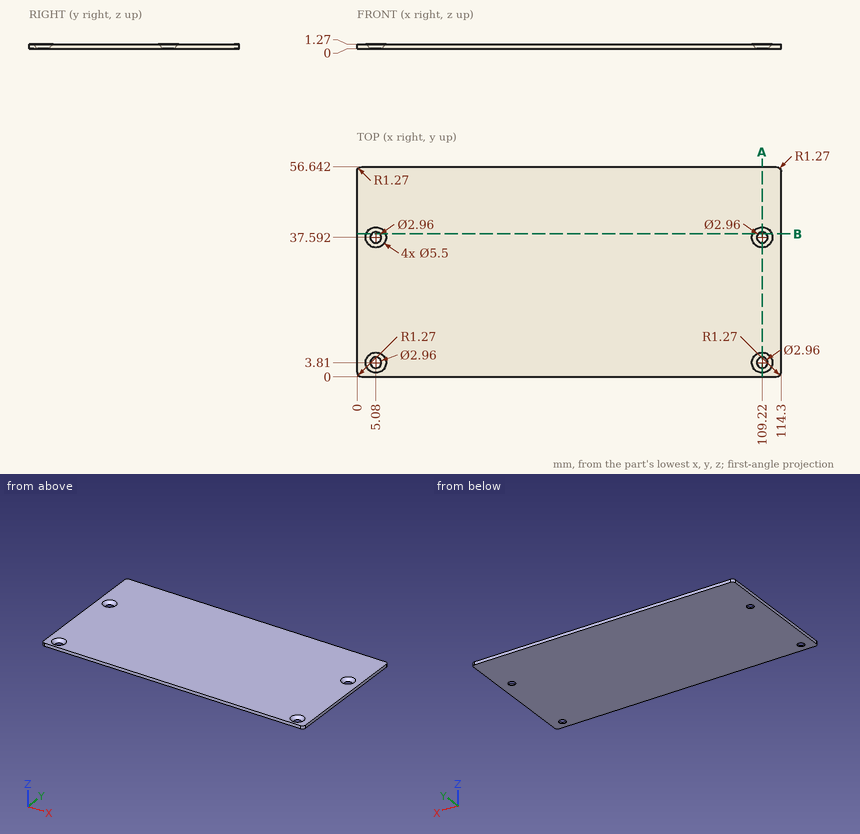
Geometry check sheet. Reference: drawing and pictorial views, mm from the part's lowest x, y, z. Round coordinates to 2 decimals unless told otherwise and drop trailing zeros. Loops run counter-clockwise (first coordinate to the right, second up) from the corner with the lowest first, then second, coordinate; pieces in that order, holes last. Notation, with made-up numbers: (-5, 70.5) -> (54, 70.5) arc R37 cw to (54, 106.5) -> close; hole circle Ø11 at (31, 87.25). An arc over 180 degrees is marked (long way). Answer as a JSON object with one key per item and string values. Group by question number.
Item 1: Cross-section at B-B, the plane y = 38.5. Count the separate pieces of the cut face and the enclosed holes in it, plus the area to 3 significant figures.
Item 2: Thickness scan on line 1 along Y through (x, z) = (107.5, 0.75); line 2 along X through (y, z) = (37, 1.1). Record the ranges inside material, lowest first.
Item 3: Depth check by flat-ended pin: pin 1 Ø10 at (x, y) = (18, 19) entering from -Z. Enter the tip coordinate at first touch or a pass-through.
Item 4: Cross-section at A-A, the plane x = 109.22. Record the cut outline in (y, z), plus the area to 3 significant figures.
Determined:
{
 "1": {"separate pieces": "3", "enclosed holes": "0", "area": "136 mm²"},
 "2": {"line 1": "y = 0 to 2.39, 5.23 to 36.17, 39.01 to 56.64", "line 2": "x = 0 to 2.57, 7.59 to 106.71, 111.73 to 114.3"},
 "3": {"pin 1": "stops at z = 0"},
 "4": {"outline": "(0, 0) -> (2.33, 0) -> (1.06, 1.27) -> (0, 1.27) -> close; (5.29, 0) -> (36.11, 0) -> (34.84, 1.27) -> (6.56, 1.27) -> close; (39.07, 0) -> (56.64, 0) -> (56.64, 1.27) -> (40.34, 1.27) -> close", "area": "61.2 mm²"}
}
